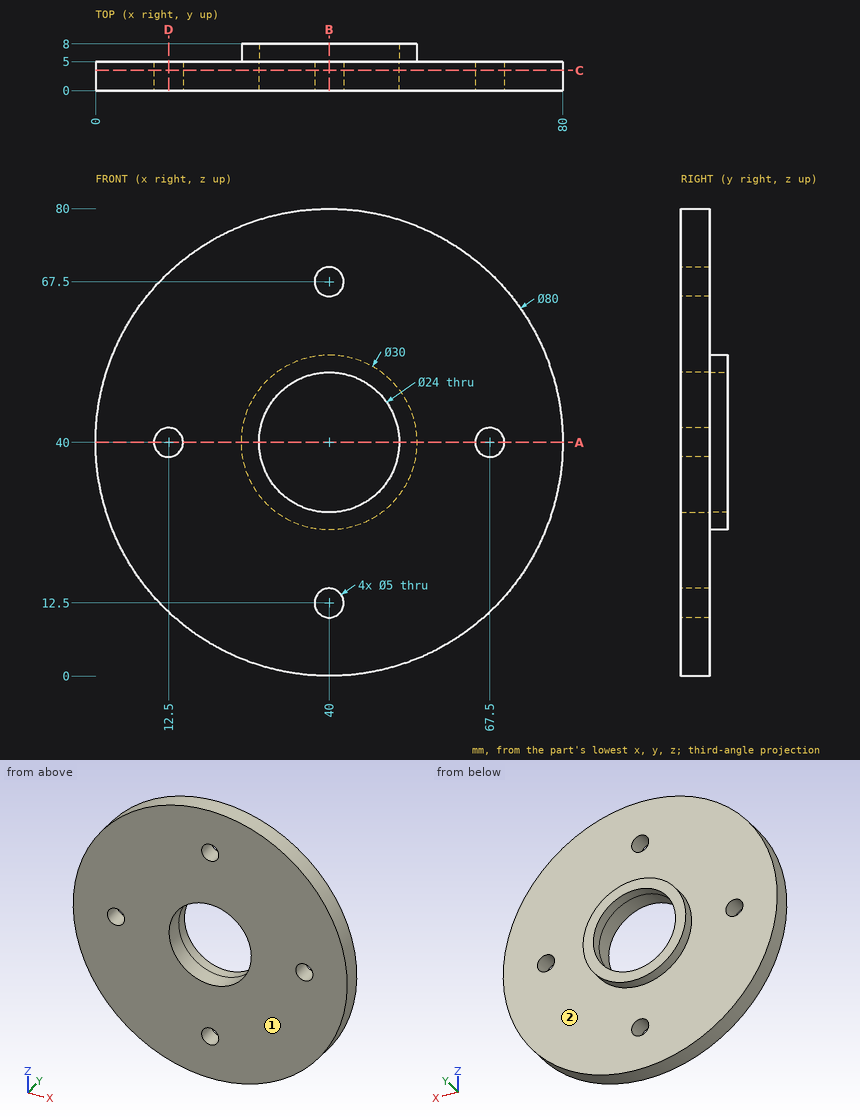
Source: three-view drawing plus pictorial views. Frame: mm from the lowest corner of the part. A direction names the side the tool comes from. Coordinates: 2 decimals unless noted, no trailing zeros. Loops run counter-clockwise (first coordinate to the right, second up) from the corner with the lowest first, then second, coordinate; pieces in that order, holes last. Notation, with made-up numbers: (39, 48.5) - (53, 48.5) arc R31 ccw to (53, 76.5) - close; hole circle Ø1 at (53, 64). An arc over 180 degrees is marked (long way). One line per question, with ' | ' between items.
1) Set-up query: the marked faces 1 and 2. Return all of +Z, -Z, +X, -X, +Y, -Y with unobstructed straight access to the full face (end or side cutting, diameter ignored); none if empty.
Report:
face 1: +Z, -Z, +X, -X, -Y | face 2: +Y
2) Section A-A, the plane z = 40. Return loops of the section in (x, y).
Report:
outline: (0, 0) - (10, 0) - (10, 5) - (0, 5) - close; (15, 0) - (28, 0) - (28, 8) - (25, 8) - (25, 5) - (15, 5) - close; (52, 0) - (65, 0) - (65, 5) - (55, 5) - (55, 8) - (52, 8) - close; (70, 0) - (80, 0) - (80, 5) - (70, 5) - close
3) First-contact query: P1, Ø8, axis at x = 64, z = 39.5, coming from the +Y side; P2, Ø1.5, axis at x = 22, y = 5.5, coming from the +Z side; P3, Ø2, axis at y = 5, z = 25.5, coming from the +X side. Flat tips, straight axial feed; report the tip coordinate or a pass-through.
Report:
P1: stops at y = 5 | P2: stops at z = 76 | P3: stops at x = 77.65
4) Section B-B, the plane x = 40. Return loops of the section in (y, z), then the cut area to 3 significant figures.
Report:
outline: (0, 0) - (5, 0) - (5, 10) - (0, 10) - close; (0, 15) - (5, 15) - (5, 25) - (8, 25) - (8, 28) - (0, 28) - close; (0, 52) - (8, 52) - (8, 55) - (5, 55) - (5, 65) - (0, 65) - close; (0, 70) - (5, 70) - (5, 80) - (0, 80) - close | area: 248 mm²
5) Line query: line 1 along X through (y, z) = (6.35, 40); line 2 along Z through (x, y) = (40.5, 7.5); line 3 along Y through (x, z) = (55.5, 47). Output: solid intervals per line, ascending.
Report:
line 1: x = 25 to 28, 52 to 55 | line 2: z = 25.01 to 28.01, 51.99 to 54.99 | line 3: y = 0 to 5
6) Section D-D, the plane x = 12.5. Return loops of the section in (y, z), then the cut area to 3 significant figures.
Report:
outline: (0, 10.95) - (5, 10.95) - (5, 37.5) - (0, 37.5) - close; (0, 42.5) - (5, 42.5) - (5, 69.05) - (0, 69.05) - close | area: 265 mm²
7) Section C-C, the plane y = 3.5. Return loops of the section in (x, z).
Report:
outline: circle Ø80 at (40, 40); hole circle Ø5 at (12.5, 40); hole circle Ø24 at (40, 40); hole circle Ø5 at (40, 12.5); hole circle Ø5 at (40, 67.5); hole circle Ø5 at (67.5, 40)
